```python
from build123d import *

# Parameters (mm, degrees)
SKETCH1_W           = 10
SKETCH1_H           = 3.175
SKETCH1_W_2         = 14
BOSS_EXTRUDE1_DEPTH = 3.175
CUT_EXTRUDE1_REACH  = 81.323


with BuildPart() as part:
    # Sketch1 → Boss-Extrude1 (new body)
    with BuildSketch(Plane.XY):
        Polygon((15, 30), (0, 0), (0, -7.175), (70, -7.175), (70, 0), (65, 30), (65, 37.175), (15, 37.175), align=None)
        with Locations((30, 31.5875)):
            Rectangle(SKETCH1_W, SKETCH1_H, mode=Mode.SUBTRACT)
        with Locations((21, -1.5875)):
            Rectangle(SKETCH1_W_2, SKETCH1_H, mode=Mode.SUBTRACT)
        with Locations((50, 31.5875)):
            Rectangle(SKETCH1_W, SKETCH1_H, mode=Mode.SUBTRACT)
        with Locations((49, -1.5875)):
            Rectangle(SKETCH1_W_2, SKETCH1_H, mode=Mode.SUBTRACT)
    extrude(amount=BOSS_EXTRUDE1_DEPTH)

    # Sketch2 → Cut-Extrude1 (cut, up to next)
    with BuildSketch(Plane.XY, mode=Mode.PRIVATE) as cut_extrude1_sk1:
        Polygon((61.611491646, 26), (65.278158313, 4), (39.440376301, 4), align=None)
    cut_extrude1_tool1 = extrude(cut_extrude1_sk1.sketch, amount=CUT_EXTRUDE1_REACH, mode=Mode.PRIVATE) & part.part
    # Sketch2 → Cut-Extrude1 (cut, up to next)
    with BuildSketch(Plane.XY, mode=Mode.PRIVATE) as cut_extrude1_sk2:
        Polygon((55.932595363, 26), (33.761480018, 4), (22.00725781, 26), align=None)
    cut_extrude1_tool2 = extrude(cut_extrude1_sk2.sketch, amount=CUT_EXTRUDE1_REACH, mode=Mode.PRIVATE) & part.part
    # Sketch2 → Cut-Extrude1 (cut, up to next)
    with BuildSketch(Plane.XY, mode=Mode.PRIVATE) as cut_extrude1_sk3:
        Polygon((17.472135955, 26), (6.472135955, 4), (29.226358163, 4), align=None)
    cut_extrude1_tool3 = extrude(cut_extrude1_sk3.sketch, amount=CUT_EXTRUDE1_REACH, mode=Mode.PRIVATE) & part.part
    add(cut_extrude1_tool1.solids().sort_by_distance((55.443342, 11.333333, 0))[0], mode=Mode.SUBTRACT)
    add(cut_extrude1_tool2.solids().sort_by_distance((37.233778, 18.666667, 0))[0], mode=Mode.SUBTRACT)
    add(cut_extrude1_tool3.solids().sort_by_distance((17.723543, 11.333333, 0))[0], mode=Mode.SUBTRACT)


solid = part.part
```
Check sheet for the modelled part. Datum: model origin and axes. Units: mm. A direction names the side the tool comes from. Give positions to 0.01 mm unless a question says otherwise; leave off trailing zeros. Loops run counter-clockwise (first coordinate to the right, second up) from the corner with the lowest first, then second, coordinate; pieces in that order, holes last. Notation, with made-up numbers: M 76,73 L 95,73 A23 cw 95,92 Z; hole C 73.5,-16 d4. An arc over 180 degrees is marked long. Answer as CSV lines item,"result".
Item 1: Scan lines: L1, parallel to Y at x = 50, z = 2.95 (3 decimals); L2, parallel to Y at x = 40.5, z = 0.25 (3 decimals); L3, parallel to X at y = 11.5, z = 2.95. Record each from-to range of solid material in increasing order.
Reply:
L1,"-7.175 to -3.175, 0 to 4, 14.478 to 20.113, 26 to 30, 33.175 to 37.175"
L2,"-7.175 to 4, 5.051 to 10.687, 26 to 37.175"
L3,"5.75 to 10.22, 25.22 to 29.75, 41.32 to 47, 64.03 to 68.08"
Item 2: Set-up check for faces 1 (the face through (21, -3.175, 2)), 2 (the face through (70, -4, 2)): record each of +Z, -Z, +X, -X, +Y, -Y from which the full face is reachable in a straight line by a thin tool's end or side.
Reply:
face 1,"+Z, -Z"
face 2,"+Z, -Z, +X, +Y, -Y"
Item 3: Sectioned sample at D-D, the plane y = 10. Enter the section's corners in (x, z) (3 decimals), then the cut area to 3 significant figures.
Reply:
outline,"M 5,0 L 9.472,0 L 9.472,3.175 L 5,3.175 Z; M 26.021,0 L 30.556,0 L 30.556,3.175 L 26.021,3.175 Z; M 39.808,0 L 45.487,0 L 45.487,3.175 L 39.808,3.175 Z; M 64.278,0 L 68.333,0 L 68.333,3.175 L 64.278,3.175 Z"
area,"59.5 mm^2"
Item 4: Sectioned sample at C-C, the plane x = 37.5. Enter the section's corners in (y, z) (3 decimals), then the cut area to 3 significant figures.
Reply:
outline,"M -7.175,0 L 7.71,0 L 7.71,3.175 L -7.175,3.175 Z; M 26,0 L 37.175,0 L 37.175,3.175 L 26,3.175 Z"
area,"82.7 mm^2"
Item 5: Sectioned sample at B-B, the plane z = 1.2. State how many separate pieces and enclosed holes the cut face has, then the cut area to 3 significant figures.
Reply:
separate pieces,"1"
enclosed holes,"7"
area,"1,600 mm^2"
Item 6: Sectioned sample at A-A, the plane y = -1.5. Enter the section's corners in (x, z) (3 decimals).
Reply:
outline,"M 0,0 L 14,0 L 14,3.175 L 0,3.175 Z; M 28,0 L 42,0 L 42,3.175 L 28,3.175 Z; M 56,0 L 70,0 L 70,3.175 L 56,3.175 Z"
Item 7: Depth check by flat-ended pin: pin 1 Ø1.6 at (y, z) = (32.5, 2) entering from +X; pin 2 Ø8 at (x, y) = (30.5, 18) entering from +Z (3 decimals). Enter the tip coordinate at first touch or a pass-through.
Reply:
pin 1,"x = 65"
pin 2,"z = 3.175"
Item 8: Draft check along Y on faces 3 (the face through (40, 37.175, 2)), 4 (the face through (45, 32, 2)), 5 (the face through (65, 34, 2)). Enter one of: pulls with the +Y half, pulls with the -Y half, needs draft (parallel to the pull), parting line crosses it, or undercut.
Reply:
face 3,"pulls with the +Y half"
face 4,"undercut"
face 5,"needs draft"
